Drawing for the job (mm, zero at the part's lowest x, y, z). Give positions to 0.01 mm unless a question says otherwise; leave off trailing zeros. Loops run counter-clockwise (first coordinate to the right, second up) from the corner with the lowest first, then second, coordinate; pieces in that order, holes last. Notation, with made-up numbers: M -14.75,26 L 36.25,26 A24 ccw 36.25,54 Z; hole C -30,70 d5. An arc over 180 degrees is marked long. Use CSV: the item, a comma, the result in double quotes. Start each with the question number.
(1) Slice it at A-A on x = 35. List the corners of the cut face in (y, z), and give its area (3 significant figures).
(2) Flat gauge pin, fed straight in: P1, Ø2, axis at x = 59.68, z = 49.25, coming from the +Y side. Where does the tip first touch, or does it go through?
(3) Slice it at C-C on y = 0.65. List the corners of the cut face in (x, z).
(4) Slice it at B-B on z = 35. List the corners of the cut face in (x, y).
(5) Slice it at D-D on x = 49. List the corners of the cut face in (y, z).
(6) Wall check: line 1 along X through (y, z) = (1.65, 35); line 2 along Z through (x, y) = (34.5, 0.5) (1 decimal); line 3 along Z through (x, y) = (48, 1.5) (1 decimal). Give the ranges that are in metal, low to high. Write a range as from..to.
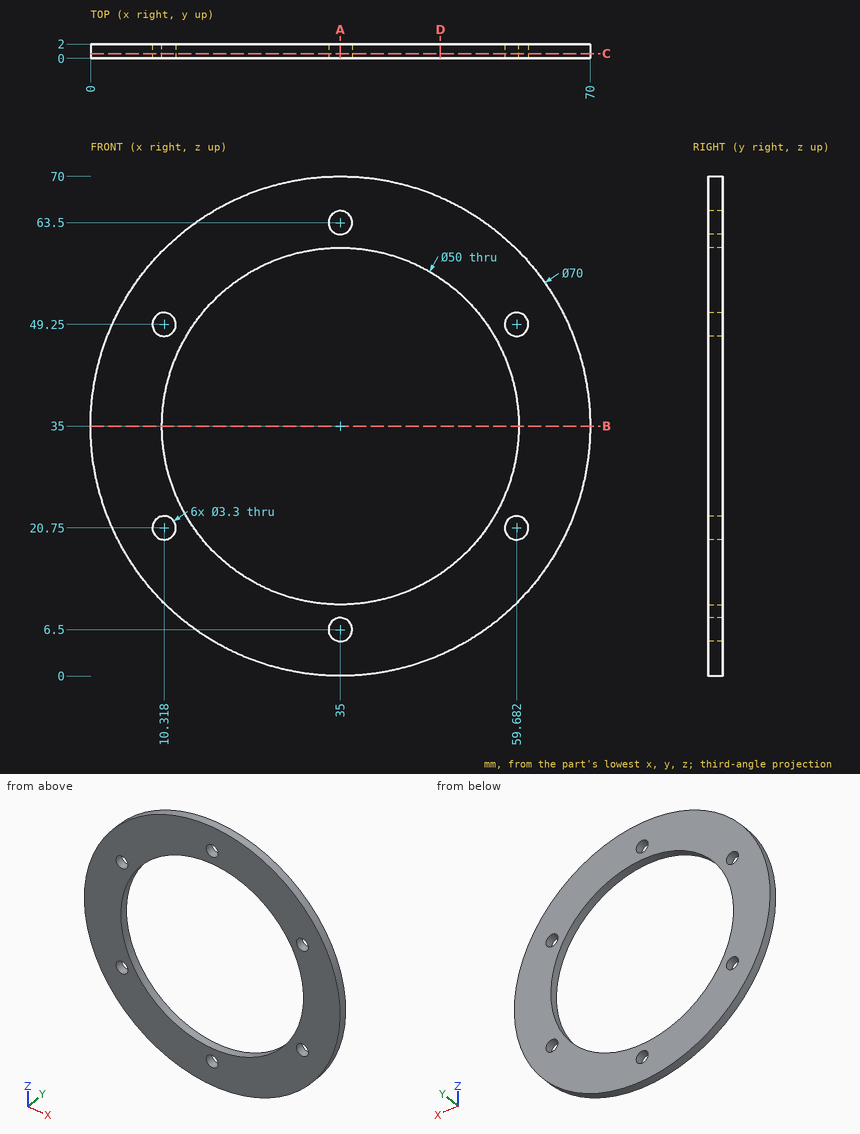
Reply:
1,outline,"M 0,0 L 2,0 L 2,4.85 L 0,4.85 Z; M 0,8.15 L 2,8.15 L 2,10 L 0,10 Z; M 0,60 L 2,60 L 2,61.85 L 0,61.85 Z; M 0,65.15 L 2,65.15 L 2,70 L 0,70 Z"
1,area,"26.8 mm^2"
2,P1,"passes through"
3,outline,"C 35,35 d70; hole C 10.32,20.75 d3.3; hole C 10.32,49.25 d3.3; hole C 35,35 d50; hole C 35,6.5 d3.3; hole C 35,63.5 d3.3; hole C 59.68,20.75 d3.3; hole C 59.68,49.25 d3.3"
4,outline,"M 0,0 L 10,0 L 10,2 L 0,2 Z; M 60,0 L 70,0 L 70,2 L 60,2 Z"
5,outline,"M 0,2.92 L 2,2.92 L 2,14.29 L 0,14.29 Z; M 0,55.71 L 2,55.71 L 2,67.08 L 0,67.08 Z"
6,line 1,"x = 0..10, 60..70"
6,line 2,"z = 0..4.9, 8.1..10, 60..61.9, 65.1..70"
6,line 3,"z = 2.5..13.6, 56.4..67.5"
